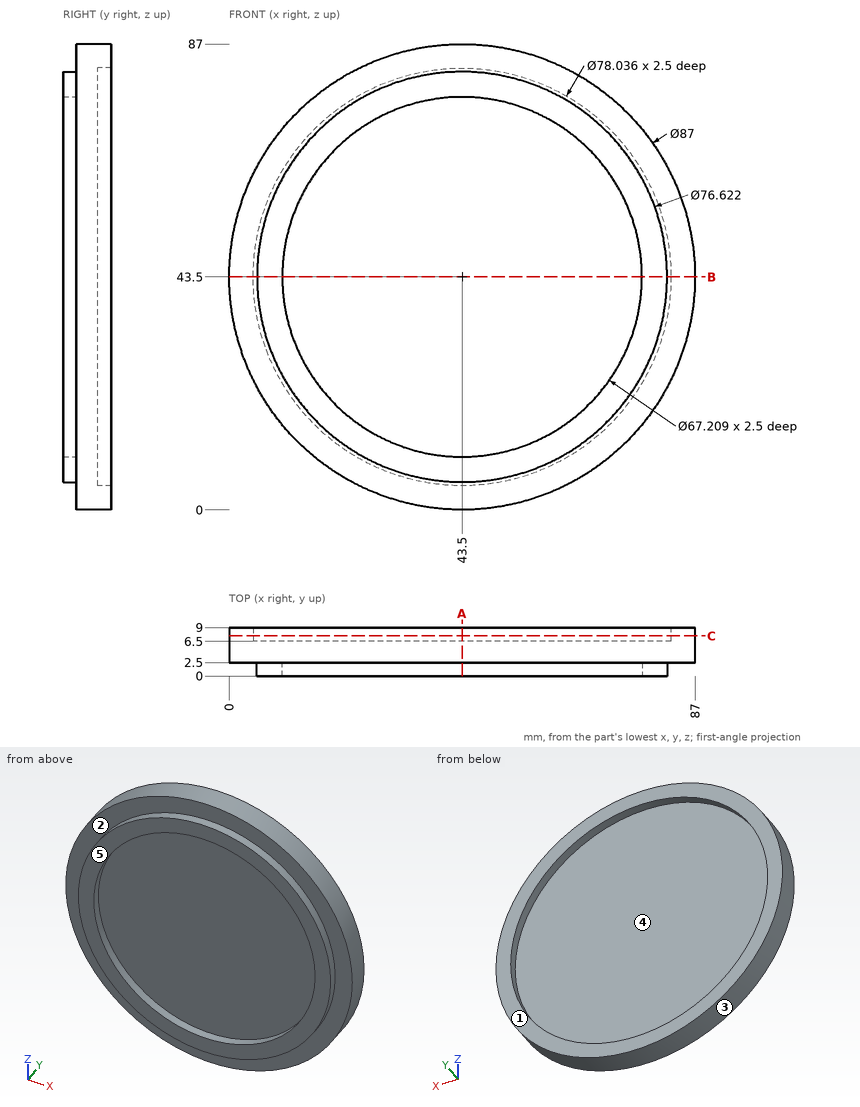
Print and shaded views of the part. All mm, measured from the part's lowest x, y and z. A direction names the side the tool comes from. Coordinates: 2 decimals unless noted, no trailing zeros. Loops run counter-clockwise (first coordinate to the right, second up) from the corner with the lowest first, then second, coordinate; pieces in that order, holes last. Notation, with made-up numbers: M 78.25,-7 L 113.25,-7 A14 cw 113.25,6 Z; hole C 16,76.25 d5. An arc over 180 degrees is marked long. Use a Markdown table: item, result. Add a question column.
Q1. Cut at A-A (x = 43.5). Write the cut outline in (y, z) (1 decimal).
Q2. Pin check, flat tips, straight feed: P1, Ø5, axis at y = 1.5, z = 20.5, coming from the -X side (1 decimal); P2, Ø4, axis at y = 5, z = 26, coming from the -X side (1 decimal); P3, Ø8, axis at x = 71.5, z = 43.5, coming from the +Y side. Stop position of each tip, or through.
Q3. Cut at C-C (y = 7.5). Write the cut outline in (x, z), and give its area (3 significant figures).
Q4. Mould opens along X. For the marked faces 3, 4 and 5 say: +X half, -X half, draft (parallel to the pull), parting line (faces both ways), or undercut.
Q5. Which spindle directions (+Z, -Z, +X, -X, +Y, -Y) get a long thin tool onto all of the face, cutting with end or side? Do the marked faces 1 and 2. Say none if no direction does.
Q6. Cut at B-B (z = 43.5). Write the cut outline in (x, y) (1 decimal), and give its area (3 significant figures).
Q7. Probe L1, parallel to Z at x = 43.5, y = 8.15; L2, parallel to Z at x = 43.5, y = 1.3 (1 decimal); L3, parallel to Y at x = 5.5, z = 59.5. List the from-to ranges inside material, lowest first.
Worked out:
| question | item | result |
|---|---|---|
| 1 | outline | M 0,5.2 L 2.5,5.2 L 2.5,0 L 9,0 L 9,4.5 L 6.5,4.5 L 6.5,82.5 L 9,82.5 L 9,87 L 2.5,87 L 2.5,81.8 L 0,81.8 L 0,77.1 L 2.5,77.1 L 2.5,9.9 L 0,9.9 Z |
| 2 | P1 | stops at x = 5.2 |
| 2 | P2 | stops at x = 2.9 |
| 2 | P3 | stops at y = 6.5 |
| 3 | outline | C 43.5,43.5 d87; hole C 43.5,43.5 d78.04 |
| 3 | area | 1,160 mm2 |
| 4 | face 3 | parting line |
| 4 | face 4 | undercut |
| 4 | face 5 | draft |
| 5 | face 1 | +Z, -Z, +X, -X, +Y |
| 5 | face 2 | -Y |
| 6 | outline | M 0,2.5 L 5.2,2.5 L 5.2,0 L 9.9,0 L 9.9,2.5 L 77.1,2.5 L 77.1,0 L 81.8,0 L 81.8,2.5 L 87,2.5 L 87,9 L 82.5,9 L 82.5,6.5 L 4.5,6.5 L 4.5,9 L 0,9 Z |
| 6 | area | 394 mm2 |
| 7 | L1 | z = 0 to 4.48, 82.52 to 87 |
| 7 | L2 | z = 5.2 to 9.9, 77.1 to 81.8 |
| 7 | L3 | y = 2.5 to 9 |
